Here's how the part is built. I have some questions about the finished solid (model axes, mm). Face numbers are marked on the shaded views. A direction names the side the tool comes from. Round coordinates to 2 decimals unless told otherwise and drop trailing zeros. Order: outer loops, then holes, each group sorted by start corner. A loop starts at its lowest first (then second) coordinate and runs counter-clockwise, first axis right, second up. Notation, with made-up numbers: (34, 75.25) -> (79, 75.25) arc R32 ccw to (79, 106.25) -> close; hole circle Ø6 at (9.5, 48). An arc over 180 degrees is marked (long way). Answer in a Markdown table with one row per item.
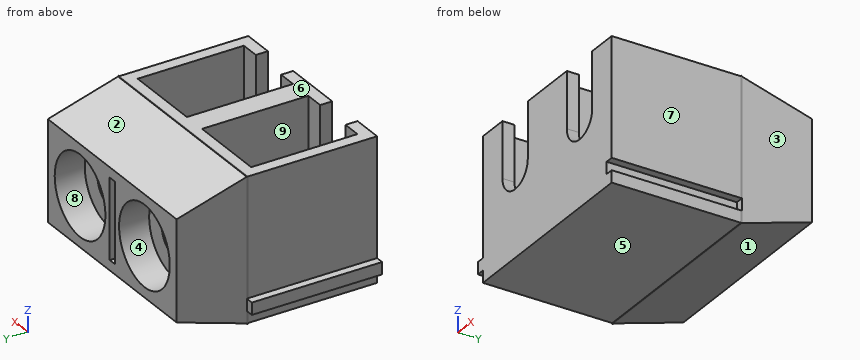
```python
from build123d import *

# Parameters (mm, degrees)
SKETCH1_W            = 10.16
SKETCH1_H            = 7.1
BOSS_EXTRUDE1_DEPTH  = 6.5
SKETCH4_W            = 10.16
SKETCH4_H            = 5
SKETCH5_W            = 3.88
SKETCH5_H            = 5.3
CUT_EXTRUDE1_DEPTH   = 6.6
SKETCH6_R            = 2
SKETCH6_W            = 0.4
SKETCH6_H            = 4
CUT_EXTRUDE2_DEPTH   = 1.5
CUT_EXTRUDE3_REACH   = 10.5
SKETCH7_R            = 1
SKETCH8_W            = 0.6
SKETCH8_H            = 6.5
CUT_EXTRUDE4_DEPTH   = 0.4
SKETCH9_W            = 0.6
SKETCH9_H            = 6.5
BOSS_EXTRUDE2_DEPTH  = 0.4
SKETCH10_W           = 7.1
SKETCH10_H           = 0.05
BOSS_EXTRUDE3_DEPTH  = 0.02
SKETCH11_W           = 10.2
SKETCH11_H           = 0.05
BOSS_EXTRUDE4_DEPTH  = 0.02
SKETCH13_W           = 0.02
SKETCH13_H           = 0.05
BOSS_EXTRUDE8_DEPTH  = 5.9
SKETCH14_W           = 0.02
SKETCH14_H           = 0.05
BOSS_EXTRUDE9_DEPTH  = 0.02
SKETCH15_W           = 0.02
SKETCH15_H           = 0.05
BOSS_EXTRUDE10_DEPTH = 10.18
SKETCH16_W           = 0.02
SKETCH16_H           = 0.05
BOSS_EXTRUDE11_DEPTH = 0.6
CUT_EXTRUDE5_REACH   = 12


with BuildPart() as part:
    # Sketch1 → Boss-Extrude1 (new body)
    with BuildSketch(Plane(origin=(0, 0, 0), x_dir=(1, 0, 0), z_dir=(0, 1, 0))):
        with Locations((-5.08, -3.55)):
            Rectangle(SKETCH1_W, SKETCH1_H)
    extrude(amount=BOSS_EXTRUDE1_DEPTH)

    # Sketch4 → section 0 of loft1
    with BuildSketch(Plane(origin=(0, 10, 0), x_dir=(1, 0, 0), z_dir=(0, 1, 0)), mode=Mode.PRIVATE) as loft1_s0:
        with Locations((-5.08, -3.6)):
            Rectangle(SKETCH4_W, SKETCH4_H)
    # loft up to a face of the part (loft1)
    loft([loft1_s0.sketch, part.faces().sort_by_distance((-5.08, 6.5, 3.55))[0]])

    # Sketch5 → Cut-Extrude1 (cut)
    with BuildSketch(Plane.XY.offset(7.1)):
        with Locations((-7.62, 3.25)):
            Rectangle(SKETCH5_W, SKETCH5_H)
        with Locations((-2.54, 3.25)):
            Rectangle(SKETCH5_W, SKETCH5_H)
    extrude(amount=-CUT_EXTRUDE1_DEPTH, mode=Mode.SUBTRACT)

    # Sketch6 → Cut-Extrude2 (cut)
    with BuildSketch(Plane(origin=(0, 10, 0), x_dir=(1, 0, 0), z_dir=(0, 1, 0))):
        with Locations((-7.62, -3.6)):
            Circle(SKETCH6_R)
        with Locations((-2.54, -3.6)):
            Circle(SKETCH6_R)
        with Locations((-5.08, -3.6)):
            Rectangle(SKETCH6_W, SKETCH6_H)
    extrude(amount=-CUT_EXTRUDE2_DEPTH, mode=Mode.SUBTRACT)

    # Sketch7 → Cut-Extrude3 (cut, up to next)
    with BuildSketch(Plane(origin=(0, 8.5, 0), x_dir=(1, 0, 0), z_dir=(0, 1, 0)), mode=Mode.PRIVATE) as cut_extrude3_sk1:
        with Locations((-7.62, -3.6)):
            Circle(SKETCH7_R)
    cut_extrude3_tool1 = extrude(cut_extrude3_sk1.sketch, amount=-CUT_EXTRUDE3_REACH, mode=Mode.PRIVATE) & part.part
    add(cut_extrude3_tool1.solids().sort_by_distance((-7.62, 8.5, 3.6))[0], mode=Mode.SUBTRACT)
    # Sketch7 → Cut-Extrude3 (cut, up to next)
    with BuildSketch(Plane(origin=(0, 8.5, 0), x_dir=(1, 0, 0), z_dir=(0, 1, 0)), mode=Mode.PRIVATE) as cut_extrude3_sk2:
        with Locations((-2.54, -3.6)):
            Circle(SKETCH7_R)
    cut_extrude3_tool2 = extrude(cut_extrude3_sk2.sketch, amount=-CUT_EXTRUDE3_REACH, mode=Mode.PRIVATE) & part.part
    add(cut_extrude3_tool2.solids().sort_by_distance((-2.54, 8.5, 3.6))[0], mode=Mode.SUBTRACT)

    # Sketch8 → Cut-Extrude4 (cut)
    with BuildSketch(Plane(origin=(0, 0, 0), x_dir=(0, 0, -1), z_dir=(1, 0, 0))):
        with Locations((-0.9, 3.25)):
            Rectangle(SKETCH8_W, SKETCH8_H)
    extrude(amount=-CUT_EXTRUDE4_DEPTH, mode=Mode.SUBTRACT)

    # Sketch9 → Boss-Extrude2 (add)
    with BuildSketch(Plane.ZY.offset(10.16)):
        with Locations((0.9, 3.25)):
            Rectangle(SKETCH9_W, SKETCH9_H)
    extrude(amount=BOSS_EXTRUDE2_DEPTH)

    # Sketch10 → Boss-Extrude3 (add)
    with BuildSketch(Plane.ZY.offset(10.16)):
        with Locations((3.55, 6.475)):
            Rectangle(SKETCH10_W, SKETCH10_H)
    extrude(amount=BOSS_EXTRUDE3_DEPTH)

    # Sketch11 → Boss-Extrude4 (add)
    with BuildSketch(Plane.XY.offset(7.1)):
        with Locations((-5.08, 6.475)):
            Rectangle(SKETCH11_W, SKETCH11_H)
    extrude(amount=BOSS_EXTRUDE4_DEPTH)

    # Sketch13 → Boss-Extrude8 (add)
    with BuildSketch(Plane(origin=(0, 0, 7.1), x_dir=(-1, 0, 0), z_dir=(0, 0, -1))):
        with Locations((-0.01, 6.475)):
            Rectangle(SKETCH13_W, SKETCH13_H)
    extrude(amount=BOSS_EXTRUDE8_DEPTH)

    # Sketch14 → Boss-Extrude9 (add)
    with BuildSketch(Plane(origin=(0, 0, 0), x_dir=(-1, 0, 0), z_dir=(0, 0, -1))):
        with Locations((10.17, 6.475)):
            Rectangle(SKETCH14_W, SKETCH14_H)
    extrude(amount=BOSS_EXTRUDE9_DEPTH)

    # Sketch15 → Boss-Extrude10 (add)
    with BuildSketch(Plane(origin=(-10.16, 0, 0), x_dir=(0, 0, -1), z_dir=(1, 0, 0))):
        with Locations((0.01, 6.475)):
            Rectangle(SKETCH15_W, SKETCH15_H)
    extrude(amount=BOSS_EXTRUDE10_DEPTH)

    # Sketch16 → Boss-Extrude11 (add)
    with BuildSketch(Plane.XY):
        with Locations((0.01, 6.475)):
            Rectangle(SKETCH16_W, SKETCH16_H)
    extrude(amount=BOSS_EXTRUDE11_DEPTH)

    # Sketch18 → Cut-Extrude5 (cut, up to next)
    with BuildSketch(Plane.XZ, mode=Mode.PRIVATE) as cut_extrude5_sk1:
        with BuildLine():
            Line((-8.62, 4.32), (-8.62, 7.92))
            ThreePointArc((-8.62, 7.92), (-7.62, 8.92), (-6.62, 7.92))
            Line((-6.62, 7.92), (-6.62, 4.32))
            ThreePointArc((-6.62, 4.32), (-7.62, 3.32), (-8.62, 4.32))
        make_face()
    cut_extrude5_tool1 = extrude(cut_extrude5_sk1.sketch, amount=-CUT_EXTRUDE5_REACH, mode=Mode.PRIVATE) & part.part
    add(cut_extrude5_tool1.solids().sort_by_distance((-7.62, 0, 6.12))[0], mode=Mode.SUBTRACT)
    # Sketch18 → Cut-Extrude5 (cut, up to next)
    with BuildSketch(Plane.XZ, mode=Mode.PRIVATE) as cut_extrude5_sk2:
        with BuildLine():
            Line((-3.54, 4.3), (-3.54, 7.9))
            ThreePointArc((-3.54, 7.9), (-2.54, 8.9), (-1.54, 7.9))
            Line((-1.54, 7.9), (-1.54, 4.3))
            ThreePointArc((-1.54, 4.3), (-2.54, 3.3), (-3.54, 4.3))
        make_face()
    cut_extrude5_tool2 = extrude(cut_extrude5_sk2.sketch, amount=-CUT_EXTRUDE5_REACH, mode=Mode.PRIVATE) & part.part
    add(cut_extrude5_tool2.solids().sort_by_distance((-2.54, 0, 6.1))[0], mode=Mode.SUBTRACT)


solid = part.part
```
1. For the marked faces 5, 6, 7, 8 and 9, which set-ups out of +Z, -Z, +X, -X, +Y, -Y let a thin tool reach every point of the face, with its end or its side?
Numbers:
| item | result |
|---|---|
| face 5 | -Z, +X, -X, -Y |
| face 6 | +Z, +X, -X, -Y |
| face 7 | +Z, -Z, +X, -Y |
| face 8 | +Y |
| face 9 | +Z |
2. Please list where these lines run through material, in increasing order: line 1 along X through (y, z) = (8.9, 3.6); line 2 along X through (y, z) = (0.75, 5); line 3 along X through (y, z) = (1.5, 0.75).
Numbers:
| item | result |
|---|---|
| line 1 | x = -10.16 to -9.62, -5.62 to -5.28, -4.88 to -4.54, -0.54 to 0 |
| line 2 | x = -10.16 to -9.56, -5.68 to -4.48, -0.6 to 0 |
| line 3 | x = -10.56 to -9.56, -5.68 to -4.48, -0.6 to -0.4 |
3. For pin 1 Ø2.5 at (x, z) = (-7.62, 3.6) entering from +Y; pin 2 Ø0.7 at (y, z) = (0.5, 5) entering from -X; pin 3 Ø4.5 at (x, y) = (-8, 4) entering from +Z, each with a flat end and sliding along its axis, tell me the tip position at first contact or that it passes through.
Numbers:
| item | result |
|---|---|
| pin 1 | stops at y = 8.5 |
| pin 2 | stops at x = -10.16 |
| pin 3 | stops at z = 7.1 |
4. We'd pull the mould along Z, two halves only. Please class the marked faces 1, 2, 3 and 4: released by +Z, released by -Z, zero draft, split by the parting line, or undercut.
Numbers:
| item | result |
|---|---|
| face 1 | released by -Z |
| face 2 | released by +Z |
| face 3 | zero draft |
| face 4 | undercut |
5. Suppose I cut it at D-D on z = 3.6. State how many separate pieces and enclosed holes the cut face has, then the cut area to 3 significant figures.
Numbers:
| item | result |
|---|---|
| separate pieces | 3 |
| enclosed holes | 0 |
| area | 35.8 mm2 |
6. Suppose I cut it at B-B on y = 2.25. Write out the boundary of the cut face in (x, z).
Numbers:
| item | result |
|---|---|
| outline | (-10.56, 0.6) -> (-10.16, 0.6) -> (-10.16, 0) -> (0, 0) -> (0, 0.6) -> (-0.4, 0.6) -> (-0.4, 1.2) -> (0, 1.2) -> (0, 7.1) -> (-0.6, 7.1) -> (-0.6, 0.5) -> (-4.48, 0.5) -> (-4.48, 7.1) -> (-5.68, 7.1) -> (-5.68, 0.5) -> (-9.56, 0.5) -> (-9.56, 7.1) -> (-10.16, 7.1) -> (-10.16, 1.2) -> (-10.56, 1.2) -> close |
